Model file for the job. Use its own axes, mm. A direction names the side the tool comes from. Give positions to 0.01 mm unless a question says otherwise; leave off trailing zeros. Order: outer loops, then holes, each group sorted by start corner. A loop starts at its lowest first (then second) coordinate and runs counter-clockwise, first axis right, second up. Notation, with made-up numbers: (-15, 64) - (33, 64) arc R10 cw to (33, 72) - close; hole circle Ø7 at (6.5, 36). An arc over 180 degrees is marked (long way). Return JSON: item names as keys, results as strings. Group by question number.
from build123d import *

# Parameters (mm, degrees)
SKETCH1_W               = 100
SKETCH1_H               = 20
BOSS_EXTRUDE1_DEPTH     = 12
SKETCH2_W               = 35
SKETCH2_H               = 20
BOSS_EXTRUDE3_DEPTH     = 15
SKETCH3_W               = 35
SKETCH3_H               = 15
BOSS_EXTRUDE4_DEPTH     = 65
FILLET1_R               = 10
CHAMFER1_SIZE           = 15
SKETCH4_R               = 10
CUT_EXTRUDE1_DEPTH      = 65
CUT_EXTRUDE1_DEPTH_BACK = 65
M5_TAPPED_HOLE1_D       = 4.2
M5_TAPPED_HOLE1_DEPTH   = 10
M5_TAPPED_HOLE1_TIP     = 1.2618073
SKETCH7_R               = 2.75
CUT_EXTRUDE2_DEPTH      = 65


with BuildPart() as part:
    # Sketch1 → Boss-Extrude1 (new body)
    with BuildSketch(Plane.XY):
        Rectangle(SKETCH1_W, SKETCH1_H)
    extrude(amount=BOSS_EXTRUDE1_DEPTH)

    # Sketch2 → Boss-Extrude3 (add)
    with BuildSketch(Plane(origin=(0, 0, 0), x_dir=(-1, 0, 0), z_dir=(0, 0, -1))):
        with Locations((-19, 0)):
            Rectangle(SKETCH2_W, SKETCH2_H)
    extrude(amount=BOSS_EXTRUDE3_DEPTH)

    # Sketch3 → Boss-Extrude4 (add)
    with BuildSketch(Plane(origin=(0, 0, -15), x_dir=(-1, 0, 0), z_dir=(0, 0, -1))):
        with Locations((-19, 0)):
            Rectangle(SKETCH3_W, SKETCH3_H)
    extrude(amount=BOSS_EXTRUDE4_DEPTH)

    # Fillet1
    fillet1_edges = [part.edges().sort_by_distance(p)[0] for p in [
        (1.5, 0, 0),
    ]]
    fillet(fillet1_edges, radius=FILLET1_R)

    # Chamfer1
    chamfer1_edges = [part.edges().sort_by_distance(p)[0] for p in [
        (1.5, 0, -80),
    ]]
    chamfer(chamfer1_edges, length=CHAMFER1_SIZE)

    # Sketch4 → Cut-Extrude1 (cut, two sides)
    with BuildSketch(Plane(origin=(0, 7.5, 0), x_dir=(1, 0, 0), z_dir=(0, 1, 0))) as cut_extrude1_sk:
        with Locations((19, 15)):
            Circle(SKETCH4_R)
        with Locations((19, 55)):
            Circle(SKETCH4_R)
    extrude(amount=CUT_EXTRUDE1_DEPTH, mode=Mode.SUBTRACT)
    extrude(cut_extrude1_sk.sketch, amount=-CUT_EXTRUDE1_DEPTH_BACK, mode=Mode.SUBTRACT)

    # M5 Tapped Hole1
    with Locations(Plane(origin=(36.5, 0, 0), x_dir=(0, 0, -1), z_dir=(1, 0, 0))):
        with Locations((72, 0), (37, 0)):
            Hole(M5_TAPPED_HOLE1_D / 2, depth=M5_TAPPED_HOLE1_DEPTH)
            with Locations((0, 0, -(M5_TAPPED_HOLE1_DEPTH + M5_TAPPED_HOLE1_TIP / 2))):  # 118° drill point
                Cone(0, M5_TAPPED_HOLE1_D / 2, M5_TAPPED_HOLE1_TIP, mode=Mode.SUBTRACT)

    # Sketch7 → Cut-Extrude2 (cut)
    with BuildSketch(Plane(origin=(0, 0, 0), x_dir=(-1, 0, 0), z_dir=(0, 0, -1))):
        with Locations((44, 0)):
            Circle(SKETCH7_R)
        with Locations((-44, 0)):
            Circle(SKETCH7_R)
    extrude(amount=-CUT_EXTRUDE2_DEPTH, mode=Mode.SUBTRACT)


solid = part.part
(1) Slice it at B-B (z = 1.5). Give the cut face in (x, y).
(2) 3-axis set-ups, long thin cutter, end or side, ignore diameter. For faces 5 (the face through (5, 9, -15)), 6 (the face through (41.7, -2.1, 0)), 7 (the face through (5, -9, -15)), 8 (the face through (1.5, 0, -37)): which of +Z, -Z, +X, -X, +Y, -Y reach the whole face in a straight line?
(3) Slice it at D-D (x = 44). Give the cut face in (y, z).
(4) Drill centre lines: L1, parallel to Z at x = 29.5, y = 0; L2, parallel to Z at x = 19, y = -0.75; L3, parallel to X at y = 4.5, z = -14.5. Where is each one in solid material? Low to high.
(5) Slice it at A-A (x = 19). Give the cut face in (y, z), and give its area (3 significant figures).
(6) Pull direction Z, two halves, no side cores. Call faces 1 (the face through (33, -9, -15)), 2 (the face through (23.614, 0.105, -46.128)), 3 (the face through (31.43, 0.09, -74.1)), 4 (the face through (46.747, 0.121, 5.916)): released by +Z, released by -Z, zero draft, split by the parting line, or undercut.
(7) Slice it at C-C (y = 4.75). Give the cut face in (x, z), and give its area (3 significant figures).
(8) Drop flat-ended pins along their axis: pin 1 Ø10 at (y, z) = (-4, -28) entering from +X; pin 2 Ø1.2 at (x, y) = (4, 8.5) entering from -Z; pin 3 Ø4 at (x, z) = (7, -33) entering from -Y. Give the stop position or say it passes through.
Result set:
{
 "1": {"outline": "(-50, -10) - (50, -10) - (50, 10) - (-50, 10) - close; hole circle Ø5.5 at (-44, 0); hole circle Ø5.5 at (44, 0)"},
 "2": {"face 5": "-Z, +X, -X, +Y", "face 6": "-Z, +X, +Y, -Y", "face 7": "-Z, +X, -X, -Y", "face 8": "-Z, -X, +Y, -Y"},
 "3": {"outline": "(-10, 0) - (-2.75, 0) - (-2.75, 12) - (-10, 12) - close; (2.75, 0) - (10, 0) - (10, 12) - (2.75, 12) - close"},
 "4": {"L1": "z = -80 to -74.1, -69.9 to -39.1, -34.9 to 12", "L2": "z = -80 to -65, -45 to -25, -5 to 12", "L3": "x = 1.5 to 9.01, 28.99 to 36.5"},
 "5": {"outline": "(-10, -5) - (10, -5) - (10, 12) - (-10, 12) - close; (-7.5, -80) - (7.5, -80) - (7.5, -65) - (-7.5, -65) - close; (-7.5, -45) - (7.5, -45) - (7.5, -25) - (-7.5, -25) - close", "area": "865 mm²"},
 "6": {"face 1": "released by -Z", "face 2": "undercut", "face 3": "undercut", "face 4": "zero draft"},
 "7": {"outline": "(-50, 0) - (-8.5, 0) arc R10 cw to (1.5, -10) - (1.5, -65) - (16.5, -80) - (36.5, -80) - (36.5, 0) - (50, 0) - (50, 12) - (-50, 12) - close; hole circle Ø20 at (19, -55); hole circle Ø20 at (19, -15)", "area": "3,280 mm²"},
 "8": {"pin 1": "stops at x = 36.5", "pin 2": "stops at z = -15", "pin 3": "stops at y = -7.5"}
}
